```python
from build123d import *

# Parameters (mm, degrees)
F1_DEPTH = 5
F2_W     = 10.2
F2_H     = 10.2
F3_DEPTH = 25
F5_DEPTH = 50


with BuildPart() as f1:
    # F0 (on Top) → F1 (new body)
    with BuildSketch(Plane.XY):
        with BuildLine():
            Line((0, 25), (-25, 25))
            Line((-25, 25), (-25, -25))
            Line((-25, -25), (25, -25))
            Line((25, -25), (25, 0))
            ThreePointArc((25, 0), (17.67767, 17.67767), (0, 25))
        make_face()
    extrude(amount=F1_DEPTH)

    # F2 (on face) → F3 (join)
    with BuildSketch(Plane.XY.offset(5)):
        Polygon((-24.2, -13.2), (-24.2, 25), (-25, 25), (-25, -25), (25, -25), (25, -24.2), (-13.2, -24.2), (-13.2, -14), (25, -14), (25, -13.2), (-13.2, -13.2), (-13.2, 25), (-14, 25), (-14, -13.2), align=None)
        with Locations((-19.1, -19.1)):
            Rectangle(F2_W, F2_H, mode=Mode.SUBTRACT)
    extrude(amount=F3_DEPTH)

    # F4 (on face) → F5 (join)
    with BuildSketch(Plane(origin=(0, 25, 0), x_dir=(-1, 0, 0), z_dir=(0, 1, 0))):
        with BuildLine():
            Line((13.2, 30), (14, 30))
            ThreePointArc((14, 30), (12.634315, 30.565685), (13.2, 29.2))
            Line((13.2, 29.2), (13.2, 30))
        make_face()
    extrude(amount=-F5_DEPTH)


solid = f1.part
```
Read the model definition and answer for the solid it produces. Units are mm, in the model's axes. A direction names the side the tool comes from. Round coordinates to 2 decimals unless told otherwise and drop trailing zeros. Write each loop counter-clockwise with the first axis right and the second up, starting at its lowest first coordinate (ties: lowest second). Pieces come first, ordered by that corner, then holes. Notation, with made-up numbers: M 18,-25.5 L 33,-25.5 A18 cw 33,-9.5 Z; hole C 84.25,-8.75 d5. An arc over 180 degrees is marked long. One line per item, written item: value.
Q1. Find section A-A on y = 20. Write down the section's boundary in (x, z), plus the area to 3 significant figures.
Data:
outline: M -25,0 L 15,0 L 15,5 L -13.2,5 L -13.2,29.2 A0.8 ccw long -14,30 L -14,5 L -24.2,5 L -24.2,30 L -25,30 Z
area: 242 mm2
Q2. Which of the six approach directions +Z, -Z, +X, -X, +Y, -Y give full straight-line access (tool end or side, diameter ignored) to faces 4 (the flat face through (-24.2, 6, 17)), 5 (the flat face through (-24.8, 0.1, 30)), 6 (the flat face through (-13.2, -19, 17))?
Data:
face 4: +Z, +Y
face 5: +Z, -X, +Y, -Y
face 6: +X
Q3. Straight lines are drawn through the part: line 1 (Y direction, x = 19.5, z = 7); line 2 (Z direction, x = 21.5, y = 5). For each, find the intervals that lie inside material, in ascending order. Write a range as [from, to].
Data:
line 1: [-25, -24.2], [-14, -13.2]
line 2: [0, 5]
Q4. For a pull along X with two mould halves and no side action, classify faces 1 (the flat face through (-14, -19, 17)), 2 (the cylindrical face through (-12.65, 0.35, 30.58)), 3 (the flat face through (-25, 0, 15)) as +X half, -X half, draft (parallel to the pull), parting line (faces both ways), or undercut.
Data:
face 1: undercut
face 2: parting line
face 3: -X half
Q5. Flat-ended cylindrical pins translate along their axes: pin 1 Ø12 at (y, z) = (-5, 15.5) entering from +X; pin 2 Ø8 at (x, y) = (0, -4.5) entering from +Z; pin 3 Ø8 at (x, y) = (12.5, -10) entering from +Z. Find the tip coordinate at first contact, or state that the pin passes through.
Data:
pin 1: x = -13.2
pin 2: z = 5
pin 3: z = 30
Q6. Find section D-D on z = 3.5. Write down the section's boundary in (x, y), plus the area to 3 significant figures.
Data:
outline: M -25,-25 L 25,-25 L 25,0 A25 ccw 0,25 L -25,25 Z
area: 2,370 mm2
Q7. Find section C-C on x = -19.5. Write down the section's boundary in (y, z).
Data:
outline: M -25,0 L 25,0 L 25,5 L -13.2,5 L -13.2,30 L -14,30 L -14,5 L -24.2,5 L -24.2,30 L -25,30 Z
Q8. Find section B-B on z = 18. Write down the section's boundary in (x, y), plus the area to 3 significant figures.
Data:
outline: M -25,-25 L 25,-25 L 25,-24.2 L -13.2,-24.2 L -13.2,-14 L 25,-14 L 25,-13.2 L -13.2,-13.2 L -13.2,25 L -14,25 L -14,-13.2 L -24.2,-13.2 L -24.2,25 L -25,25 Z; hole M -24.2,-24.2 L -14,-24.2 L -14,-14 L -24.2,-14 Z
area: 157 mm2
